Build history of the part. All positions in model axes, mm. A direction names the side the tool comes from. Give positions to 0.01 mm unless a question says otherwise; leave off trailing zeros. Order: outer loops, then holes, each group sorted by start corner. A loop starts at its lowest first (then second) coordinate and runs counter-clockwise, first axis right, second up. Notation, with made-up numbers: (83, -14.75) - (98, -14.75) arc R10 ccw to (98, 0.25) - close; hole circle Ø3 at (37, -30.5). An arc over 180 degrees is marked (long way). Use a Markdown table: item, result.
from build123d import *

# Parameters (mm, degrees)
BOSS_EXTRUDE1_DEPTH = 2
BOSS_EXTRUDE2_DEPTH = 8
SKETCH7_W           = 20
SKETCH7_H           = 16
CUT_EXTRUDE4_DEPTH  = 1
SKETCH8_W           = 23.5
SKETCH8_H           = 10
CUT_EXTRUDE5_DEPTH  = 205.156097213
SKETCH9_W           = 10
SKETCH9_H           = 23.5
CUT_EXTRUDE6_DEPTH  = 197.517261647
SKETCH16_W          = 16
SKETCH16_H          = 4
CUT_EXTRUDE7_DEPTH  = 10
SKETCH17_W          = 12
SKETCH17_H          = 4
CUT_EXTRUDE8_DEPTH  = 115.37923137
SKETCH18_W          = 14.430433489
SKETCH18_H          = 4
CUT_EXTRUDE9_DEPTH  = 9


with BuildPart() as part:
    # Sketch1 → Boss-Extrude1 (new body)
    with BuildSketch(Plane(origin=(0, 0, 0), x_dir=(1, 0, 0), z_dir=(0, 1, 0))):
        Polygon((23, -85.533895191), (23, -95.533895191), (23, -158.033895191), (46.5, -158.033895191), (46.5, -95.533895191), (66.5, -95.533895191), (66.5, -75.533895191), (129, -75.533895191), (129, -52.033895191), (66.5, -52.033895191), (56.5, -52.033895191), (56.5, -85.533895191), align=None)
    extrude(amount=BOSS_EXTRUDE1_DEPTH)

    # Sketch2 → Boss-Extrude2 (add)
    with BuildSketch(Plane(origin=(0, 2, 0), x_dir=(1, 0, 0), z_dir=(0, 1, 0))):
        Polygon((56.5, -52.033895191), (61.5, -52.033895191), (61.5, -90.533895191), (23, -90.533895191), (23, -85.533895191), (56.5, -85.533895191), align=None)
    extrude(amount=BOSS_EXTRUDE2_DEPTH)

    # Sketch7 → Cut-Extrude4 (cut)
    with BuildSketch(Plane(origin=(0, 2, 0), x_dir=(1, 0, 0), z_dir=(0, 1, 0))):
        with Locations((119, -63.783895191)):
            Rectangle(SKETCH7_W, SKETCH7_H)
    extrude(amount=-CUT_EXTRUDE4_DEPTH, mode=Mode.SUBTRACT)

    # Sketch8 → Cut-Extrude5 (cut, through all)
    with BuildSketch(Plane(origin=(0, 2, 0), x_dir=(1, 0, 0), z_dir=(0, 1, 0))):
        with Locations((34.75, -153.033895191)):
            Rectangle(SKETCH8_W, SKETCH8_H)
    extrude(amount=-CUT_EXTRUDE5_DEPTH, mode=Mode.SUBTRACT)

    # Sketch9 → Cut-Extrude6 (cut, through all)
    with BuildSketch(Plane(origin=(0, 2, 0), x_dir=(1, 0, 0), z_dir=(0, 1, 0))):
        with Locations((124, -63.783895191)):
            Rectangle(SKETCH9_W, SKETCH9_H)
    extrude(amount=-CUT_EXTRUDE6_DEPTH, mode=Mode.SUBTRACT)

    # Sketch11 → Loft3 section 0
    with BuildSketch(Plane.XY.offset(90.533895191)):
        with BuildLine():
            Line((46.5, 2), (46.5, 10))
            Line((46.5, 10), (23, 10))
            Line((23, 10), (23, 2))
            Line((23, 2), (46.5, 2))
        make_face()
    # Sketch13 → Loft3 section 1
    with BuildSketch(Plane.XY.offset(148.033895191)):
        with BuildLine():
            Line((23, 2), (23, 2.2))
            Line((23, 2.2), (46.5, 2.2))
            Line((46.5, 2.2), (46.5, 2))
            Line((46.5, 2), (23, 2))
        make_face()
    loft3 = loft()

    # Sketch16 → Cut-Extrude7 (cut)
    with BuildSketch(Plane.XY.offset(148.033895191)):
        with Locations((34.75, 3.2)):
            Rectangle(SKETCH16_W, SKETCH16_H)
    cut_extrude7 = extrude(amount=-CUT_EXTRUDE7_DEPTH, mode=Mode.SUBTRACT)

    # Mirror2: Loft3, Cut-Extrude7 across plane
    add(loft3.mirror(Plane(origin=(-14.516947595, 0, 14.516947595), x_dir=(0.7071067811865507, 0, 0.7071067811865444), z_dir=(-0.7071067811865446, 0, 0.7071067811865506))))
    add(cut_extrude7.mirror(Plane(origin=(-14.516947595, 0, 14.516947595), x_dir=(0.7071067811865507, 0, 0.7071067811865444), z_dir=(-0.7071067811865446, 0, 0.7071067811865506))), mode=Mode.SUBTRACT)

    # Sketch17 → Cut-Extrude8 (cut, through all)
    with BuildSketch(Plane(origin=(54.266947595, 0, 54.266947595), x_dir=(0.7071067811865475, 0, -0.7071067811865477), z_dir=(0.7071067811865477, 0, 0.7071067811865475))):
        with Locations((-20.530064174, 4)):
            Rectangle(SKETCH17_W, SKETCH17_H)
    extrude(amount=CUT_EXTRUDE8_DEPTH, mode=Mode.SUBTRACT)

    # Sketch18 → Cut-Extrude9 (cut, symmetric)
    with BuildSketch(Plane(origin=(-14.516947595, 0, 14.516947595), x_dir=(0.7071067811865446, 0, 0.7071067811865505), z_dir=(-0.7071067811865505, 0, 0.7071067811865446))):
        with Locations((106.719415005, 4)):
            Rectangle(SKETCH18_W, SKETCH18_H)
    extrude(amount=CUT_EXTRUDE9_DEPTH, both=True, mode=Mode.SUBTRACT)


solid = part.part
1) Slice it at B-B (z = 70). Write the cut outline in (x, y), and give its area (3 significant figures).
Computed:
| item | result |
|---|---|
| outline | (56.5, 0) - (119, 0) - (119, 1) - (109, 1) - (109, 3.56) - (61.5, 10) - (56.5, 10) - close |
| area | 382 mm² |
2) Two-plate mould, pull along X, no slides. Class faces 1 (the flat face through (84.264, 6.912, 63.948)), 2 (the flat face through (35, 2, 138.034)), 3 (the flat face through (23, 4, 110)), 4 (the flat face through (35, 1, 148.034)): +X half, -X half, draft (parallel to the pull), parting line (faces both ways), or undercut.
Computed:
| item | result |
|---|---|
| face 1 | +X half |
| face 2 | undercut |
| face 3 | -X half |
| face 4 | draft |
3) Slice it at C-C (y = 8.75). Write the cut outline in (x, z).
Computed:
| item | result |
|---|---|
| outline | (23, 85.53) - (56.5, 85.53) - (56.5, 52.03) - (70.71, 52.03) - (70.71, 75.53) - (61.5, 75.53) - (61.5, 90.53) - (46.5, 90.53) - (46.5, 99.75) - (23, 99.75) - close |
4) Tool access for faces 5 (the flat face through (52, 8, 90.534)), 6 (the flat face through (35, 1.2, 143)), 7 (the flat face through (49.78, 3.97, 87.3)), 8 (the flat face through (56.5, 5, 69)): list every direction of +Z, -Z, +X, -X, +Y, -Y with a clear straight run to the whole face (end or side of a thin tool).
Computed:
| item | result |
|---|---|
| face 5 | +Z, +X, +Y |
| face 6 | +Z, +Y |
| face 7 | -Z, +X |
| face 8 | -Z, -X, +Y, -Y |
5) Slice it at A-A (x = 41.5). Write the cut outline in (y, z).
Computed:
| item | result |
|---|---|
| outline | (0, 85.53) - (10, 85.53) - (10, 90.53) - (3.56, 138.03) - (1.2, 138.03) - (1.2, 148.03) - (0, 148.03) - close |
6) Pin check, flat tips, straight feed: P1, Ø2.5, axis at x = 35.5, y = 2.5, coming from the +Z side; P2, Ø5, axis at y = 2, z = 119.5, coming from the +X side; P3, Ø2.5, axis at x = 52, y = 6, coming from the +Z side; P4, Ø5, axis at y = 7, z = 133.5, coming from the +X side. Stop position of each tip, or through.
Computed:
| item | result |
|---|---|
| P1 | stops at z = 138.03 |
| P2 | stops at x = 46.5 |
| P3 | stops at z = 90.53 |
| P4 | passes through |
7) Wall check: line 1 (X direction, y = 1.25, z = 138.5); line 2 (Z direction, x = 64.5, y = 3.5); line 3 (Z direction, x = 29, y = 2.5). Give the ranges that are in metal, low to high. Write a range as from..to.
Computed:
| item | result |
|---|---|
| line 1 | x = 23..26.75, 42.75..46.5 |
| line 2 | z = 52.03..75.53 |
| line 3 | z = 85.53..138.03 |
8) Slice it at D-D (x = 111). Write the cut outline in (y, z), and give its area (3 significant figures).
Computed:
| item | result |
|---|---|
| outline | (0, 52.03) - (3.29, 52.03) - (3.29, 55.78) - (1, 55.78) - (1, 71.78) - (3.29, 71.78) - (3.29, 75.53) - (0, 75.53) - close |
| area | 40.6 mm² |
